Check sheet for the modelled part. Datum: model origin and axes. Units: mm. A direction names the side the tool comes from. Round coordinates to 2 decimals unless told otherwise and drop trailing zeros. Order: outer loops, then holes, each group sorted by start corner. A loop starts at its lowest first (then second) coordinate and runs counter-clockwise, first axis right, second up.
```python
from build123d import *

# Parameters (mm, degrees)
SKETCH1_W                  = 83.2739
SKETCH1_H                  = 30.5689
PROTON_PCB_DEPTH           = 1.58115
SKETCH2_W                  = 15.481187868
SKETCH2_H                  = 5.216136306
JST_6_PIN_CONNECTORS_DEPTH = 10
SKETCH3_W                  = 2.54
SKETCH3_H                  = 25.4
BOSS_EXTRUDE1_DEPTH        = 10.668
SKETCH4_R                  = 1.4652625
CUT_EXTRUDE1_DEPTH         = 1.58115
SKETCH5_W                  = 4.572
SKETCH5_H                  = 3.556
BOSS_EXTRUDE2_DEPTH        = 1.778
SKETCH6_W                  = 17.78
SKETCH6_H                  = 6.858
BOSS_EXTRUDE3_DEPTH        = 2.794


with BuildPart() as part:
    # Sketch1 → Proton PCB (new body)
    with BuildSketch(Plane(origin=(0, 0, 0), x_dir=(1, 0, 0), z_dir=(0, 1, 0))):
        Rectangle(SKETCH1_W, SKETCH1_H)
    extrude(amount=PROTON_PCB_DEPTH)

    # Sketch2 → JST 6 pin Connectors (add)
    with BuildSketch(Plane(origin=(0, 1.58115, 0), x_dir=(1, 0, 0), z_dir=(0, 1, 0))):
        with Locations((-21.31695, 5.12445)):
            Rectangle(SKETCH2_W, SKETCH2_H)
        with Locations((-21.31695, -5.12445)):
            Rectangle(SKETCH2_W, SKETCH2_H)
    extrude(amount=JST_6_PIN_CONNECTORS_DEPTH)

    # Sketch3 → Boss-Extrude1 (add)
    with BuildSketch(Plane(origin=(0, 1.58115, 0), x_dir=(1, 0, 0), z_dir=(0, 1, 0))):
        with Locations((-32.74695, 0)):
            Rectangle(SKETCH3_W, SKETCH3_H)
    extrude(amount=BOSS_EXTRUDE1_DEPTH)

    # Sketch4 → Cut-Extrude1 (cut)
    with BuildSketch(Plane(origin=(0, 1.58115, 0), x_dir=(1, 0, 0), z_dir=(0, 1, 0))):
        with Locations((-39.4033375, 13.0508375)):
            Circle(SKETCH4_R)
        with Locations((39.4033375, 13.0508375)):
            Circle(SKETCH4_R)
        with Locations((-39.4033375, -13.0508375)):
            Circle(SKETCH4_R)
        with Locations((39.4033375, -13.0508375)):
            Circle(SKETCH4_R)
    extrude(amount=-CUT_EXTRUDE1_DEPTH, mode=Mode.SUBTRACT)

    # Sketch5 → Boss-Extrude2 (add)
    with BuildSketch(Plane.XZ):
        with Locations((-20.55495, 9.44245)):
            Rectangle(SKETCH5_W, SKETCH5_H)
        with Locations((-25.88895, 9.44245)):
            Rectangle(SKETCH5_W, SKETCH5_H)
        with Locations((-15.22095, 9.44245)):
            Rectangle(SKETCH5_W, SKETCH5_H)
        with Locations((23.60295, -2.83845)):
            Rectangle(SKETCH5_W, SKETCH5_H)
        with Locations((-15.22095, -9.44245)):
            Rectangle(SKETCH5_W, SKETCH5_H)
        with Locations((-20.55495, -9.44245)):
            Rectangle(SKETCH5_W, SKETCH5_H)
        with Locations((-25.88895, -9.44245)):
            Rectangle(SKETCH5_W, SKETCH5_H)
    extrude(amount=BOSS_EXTRUDE2_DEPTH)

    # Sketch6 → Boss-Extrude3 (add)
    with BuildSketch(Plane.XZ):
        with Locations((-2.26695, 6.77545)):
            Rectangle(SKETCH6_W, SKETCH6_H)
    extrude(amount=BOSS_EXTRUDE3_DEPTH)


solid = part.part
```
Item 1: Access from +Z, -Z, +X, -X, +Y, -Y to the whole of each face (thin tool, end or side, straight path). Record for faces 1 (the flat face through (-26, -1, 11.22)), 2 (the flat face through (-26, -1, -11.22)), 3 (the flat face through (-18.269, -1, 9)), 4 (the flat face through (-21, -1, 7.664)).
Answer:
face 1: +Z, +X, -X, -Y
face 2: -Z, +X, -X, -Y
face 3: +Z, -Z, -Y
face 4: -X, -Y
Item 2: Release check for a two-part mould opening along X. For faces 5 (the flat face through (-18.269, -1, -9)), 6 (the flat face through (-28.175, -1, -9)), 7 (the flat face through (-29.058, 7, -5)), 8 (the flat face through (-13.576, 7, 5)) record: released by +X, released by -X, zero draft, split by the parting line, or undercut.
Answer:
face 5: undercut
face 6: released by -X
face 7: undercut
face 8: released by +X
Item 3: Sectioned sample at B-B (x = 25). Record the cut outline in (y, z).
Answer:
outline: (-1.78, -4.62) - (0, -4.62) - (0, -15.28) - (1.58, -15.28) - (1.58, 15.28) - (0, 15.28) - (0, -1.06) - (-1.78, -1.06) - close
Item 4: Go/stop test with flat-tipped pins: P1, Ø0.8, axis at x = -33, y = 6.5, coming from the +Z side; P2, Ø1, axis at x = 17, z = -6.5, coming from the +Y side; P3, Ø0.5, axis at y = -0.5, z = -8.5, coming from the -X side. Record where each tip stops, or that it passes through.
Answer:
P1: stops at z = 12.7
P2: stops at y = 1.58
P3: stops at x = -28.17
Item 5: Scan lines: line 1 along Z through (x, y) = (-14.5, 9); line 2 along X through (y, z) = (2, 5.5); line 3 along Y through (x, z) = (1, -1). Record each from-to range of solid material in increasing order.
Answer:
line 1: z = -7.73 to -2.52, 2.52 to 7.73
line 2: x = -34.02 to -31.48, -29.06 to -13.58
line 3: y = 0 to 1.58
Item 6: Sectioned sample at D-D (x = -8). Record the cut outline in (y, z), and give its area (3 significant figures).
Answer:
outline: (-2.79, 3.35) - (0, 3.35) - (0, -15.28) - (1.58, -15.28) - (1.58, 15.28) - (0, 15.28) - (0, 10.2) - (-2.79, 10.2) - close
area: 67.5 mm2
Item 7: Sectioned sample at C-C (z = -6.5). Record the cut outline in (x, y).
Answer:
outline: (-41.64, 0) - (41.64, 0) - (41.64, 1.58) - (-13.58, 1.58) - (-13.58, 11.58) - (-29.06, 11.58) - (-29.06, 1.58) - (-31.48, 1.58) - (-31.48, 12.25) - (-34.02, 12.25) - (-34.02, 1.58) - (-41.64, 1.58) - close
Item 8: Sectioned sample at A-A (y = 5.5). Record the cut outline in (x, z), and give its area (3 significant figures).
Answer:
outline: (-34.02, -12.7) - (-31.48, -12.7) - (-31.48, 12.7) - (-34.02, 12.7) - close; (-29.06, -7.73) - (-13.58, -7.73) - (-13.58, -2.52) - (-29.06, -2.52) - close; (-29.06, 2.52) - (-13.58, 2.52) - (-13.58, 7.73) - (-29.06, 7.73) - close
area: 226 mm2
